from build123d import *

# Parameters (mm, degrees)
SKETCH_R        = 0.86
SKETCH_R_2      = 1.5
SKETCH_R_3      = 1.65
SKETCH_W        = 8.7
SKETCH_H        = 20.4
PAD_DEPTH       = 3
SKETCH001_R     = 0.86
SKETCH001_W     = 8.7
SKETCH001_H     = 20.4
PAD001_DEPTH    = 5.5
PAD002_DEPTH    = 36
CHAMFER_1_ANGLE = 15
CHAMFER_1_SIZE  = 29.85
CHAMFER_2_ANGLE = 15
CHAMFER_2_SIZE  = 29.85
SKETCH003_R     = 1.05
SKETCH003_W     = 20
SKETCH003_H     = 3
POCKET_DEPTH    = 3
POCKET001_DEPTH = 1


with BuildPart() as part:
    # Sketch → Pad (new body)
    with BuildSketch(Plane.XY):
        with BuildLine():
            Line((-11.3, -4), (-26, -4))
            Line((-26, -4), (-34, -4))
            ThreePointArc((-34, 4), (-38, 0), (-34, -4))
            Line((-34, 4), (-26, 4))
            Line((-26, 4), (-10, 22))
            Line((-10, 22), (10, 22))
            Line((26, 4), (10, 22))
            Line((26, 4), (34, 4))
            ThreePointArc((34, -4), (38, 0), (34, 4))
            Line((26, -4), (34, -4))
            Line((11.3, -4), (26, -4))
            Line((6, -23.75), (11.3, -4))
            Line((-6, -23.75), (6, -23.75))
            Line((-11.3, -4), (-6, -23.75))
        make_face()
        with Locations((0, 2.25)):
            Circle(SKETCH_R, mode=Mode.SUBTRACT)
        with Locations((0, -21.35)):
            Circle(SKETCH_R, mode=Mode.SUBTRACT)
        with Locations((-34, 0)):
            Circle(SKETCH_R_2, mode=Mode.SUBTRACT)
        with Locations((34, 0)):
            Circle(SKETCH_R_2, mode=Mode.SUBTRACT)
        with Locations((-22, 0)):
            Circle(SKETCH_R_3, mode=Mode.SUBTRACT)
        with Locations((-11.319468, 16)):
            Circle(SKETCH_R_3, mode=Mode.SUBTRACT)
        with Locations((11.319468, 16)):
            Circle(SKETCH_R_3, mode=Mode.SUBTRACT)
        with Locations((22, 0)):
            Circle(SKETCH_R_3, mode=Mode.SUBTRACT)
        with Locations((0, -9.55)):
            Rectangle(SKETCH_W, SKETCH_H, mode=Mode.SUBTRACT)
    extrude(amount=PAD_DEPTH)

    # Sketch001 (on Face24 of Pad) → Pad001 (join)
    with BuildSketch(Plane.XY.offset(3)):
        Polygon((-6, -23.75), (6, -23.75), (9.810633, -9.55), (6, 4.65), (-6, 4.65), (-9.810633, -9.55), align=None)
        with Locations((0, -21.35)):
            Circle(SKETCH001_R, mode=Mode.SUBTRACT)
        with Locations((0, 2.25)):
            Circle(SKETCH001_R, mode=Mode.SUBTRACT)
        with Locations((0, -9.55)):
            Rectangle(SKETCH001_W, SKETCH001_H, mode=Mode.SUBTRACT)
    extrude(amount=PAD001_DEPTH)

    # Sketch002 (on Face5 of Pad001) → Pad002 (join)
    with BuildSketch(Plane.XY.offset(3)):
        Polygon((-12, 6.65), (-12, -1.35), (-13.5, -1.35), (-13.5, 9.65), (13.5, 9.65), (13.5, -1.35), (12, -1.35), (12, 6.65), align=None)
    extrude(amount=PAD002_DEPTH)

    # Chamfer 1
    chamfer_1_edges = [part.edges().sort_by_distance(p)[0] for p in [
        (-12.75, -1.35, 39),
    ]]
    chamfer_1_side = part.faces().sort_by_distance((-12.75, -1.35, 21))[0]
    chamfer(chamfer_1_edges, length=CHAMFER_1_SIZE, angle=CHAMFER_1_ANGLE, reference=chamfer_1_side)

    # Chamfer 2
    chamfer_2_edges = [part.edges().sort_by_distance(p)[0] for p in [
        (12.75, -1.35, 39),
    ]]
    chamfer_2_side = part.faces().sort_by_distance((12.75, -1.35, 21))[0]
    chamfer(chamfer_2_edges, length=CHAMFER_2_SIZE, angle=CHAMFER_2_ANGLE, reference=chamfer_2_side)

    # Sketch003 (on Face26 of Chamfer) → Pocket (cut)
    with BuildSketch(Plane(origin=(0, 9.65, 0), x_dir=(-1, 0, 0), z_dir=(0, 1, 0))):
        with Locations((-10.25, 6)):
            Circle(SKETCH003_R)
        with Locations((-10.25, 19.5)):
            Circle(SKETCH003_R)
        with Locations((10.25, 6)):
            Circle(SKETCH003_R)
        with Locations((10.25, 19.5)):
            Circle(SKETCH003_R)
        with Locations((0, 35)):
            Rectangle(SKETCH003_W, SKETCH003_H)
    extrude(amount=-POCKET_DEPTH, mode=Mode.SUBTRACT)

    # Sketch004 (on Face41 of Pocket) → Pocket001 (cut)
    with BuildSketch(Plane(origin=(0, 0, 0), x_dir=(1, 0, 0), z_dir=(0, 0, -1))):
        Polygon((-8, 2.75), (-11.3, 4), (-6, 23.75), (6, 23.75), (11.3, 4), (8, 2.75), (6, -4.65), (-6, -4.65), align=None)
    extrude(amount=-POCKET001_DEPTH, mode=Mode.SUBTRACT)


solid = part.part
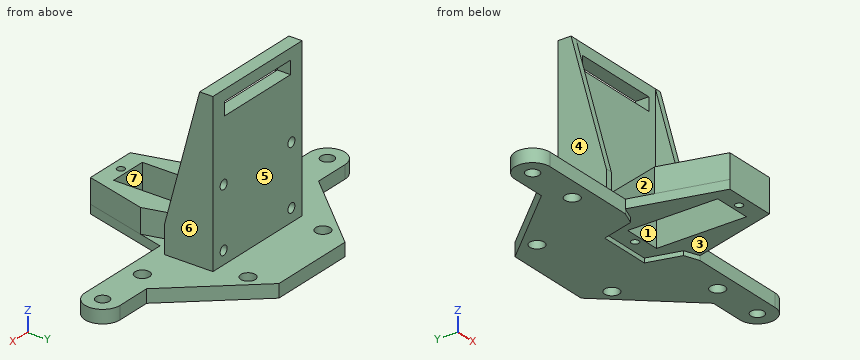
Could you check a few things on this model? Use its own coordinates, in mm. Face numbers are marked on the shaded views. A direction names the side the tool comes from. Give positions to 0.01 mm unless a question says otherwise; leave off trailing zeros. Order: outer loops, then holes, each group sorted by start corner. A loop starts at its lowest first (then second) coordinate and runs counter-clockwise, first axis right, second up. Notation, with made-up numbers: (83, 51.25) - (137, 51.25) arc R13 ccw to (137, 57.25) - close; hole circle Ø2 at (-7, -18). An arc over 180 degrees is marked (long way). Return JSON: item names as keys, results as strings. Group by question number.
Q1. Will these pins go through, and if not, where does the flat tip stop? pin 1 Ø2 at (x, y) = (0, 2.25) entering from +Z; pin 2 Ø7 at (x, y) = (2.5, -14) entering from -Z; pin 3 Ø1.2 at (x, z) = (-13, 5) entering from -Y.
Q2. Suppose I cut it at B-B, the plane y = 16. Please give me the cut outline in (x, z).
Q3. Thinking about a two-plate mould opening in X: for the marked faces 5, 6 and 7, which applies, pulls with the +X half, pulls with the -X half, needs draft (parallel to the pull), parting line crosses it, or undercut?
Q4. Suppose I cut it at D-D, the plane z = 23. Please give me the cut outline in (x, y).
Q5. Suppose I cut it at C-C, the plane y = -6. Please give me the cut outline in (x, z), and give its area (3 significant figures).
Q6. Please list where these lines run through material, in increasing order: line 1 along Y through (x, z) = (0, 5); line 2 along Z through (x, y) = (-10.25, 7.4); line 3 along X through (y, z) = (2.25, 3.5). Write a range as [from, to].
Q7. Which directions (+Z, -Z, +X, -X, +Y, -Y) give clear straight access to the entire face, cutting with the end or side of a thin tool? Please do the marked faces 1, 2, 3 and 4.
Q8. Suppose I cut it at A-A, the plane x = -22. Please give me the cut outline in (y, z), and give its area (3 significant figures).
Resolved:
{
 "1": {"pin 1": "stops at z = 8.5", "pin 2": "stops at z = 1", "pin 3": "stops at y = -1.35"},
 "2": {"outline": "(-15.33, 0) - (-12.97, 0) - (-12.97, 3) - (-15.33, 3) - close; (-9.67, 0) - (9.67, 0) - (9.67, 3) - (-9.67, 3) - close; (12.97, 0) - (15.33, 0) - (15.33, 3) - (12.97, 3) - close"},
 "3": {"face 5": "needs draft", "face 6": "pulls with the +X half", "face 7": "undercut"},
 "4": {"outline": "(-13.5, 2.36) - (-12, 2.36) - (-12, 6.65) - (12, 6.65) - (12, 2.36) - (13.5, 2.36) - (13.5, 9.65) - (-13.5, 9.65) - close"},
 "5": {"outline": "(-10.76, 1) - (-4.35, 1) - (-4.35, 8.5) - (-8.86, 8.5) - (-8.86, 3) - (-10.76, 3) - close; (4.35, 1) - (10.76, 1) - (10.76, 3) - (8.86, 3) - (8.86, 8.5) - (4.35, 8.5) - close", "area": "75.2 mm2"},
 "6": {"line 1": "y = [-23.75, -22.21], [-20.49, -19.75], [0.65, 1.39], [3.11, 4.65], [6.65, 9.65]", "line 2": "z = [0, 4.95], [7.05, 18.45], [20.55, 39]", "line 3": "x = [-13.5, -12], [-6.64, -0.86], [0.86, 6.64], [12, 13.5]"},
 "7": {"face 1": "+Z, -Z", "face 2": "+Z", "face 3": "-Z, -Y", "face 4": "+Z, -X, +Y, -Y"},
 "8": {"outline": "(-4, 0) - (-1.65, 0) - (-1.65, 3) - (-4, 3) - close; (1.65, 0) - (8.5, 0) - (8.5, 3) - (1.65, 3) - close", "area": "27.6 mm2"}
}
